Input: part model. Units: mm. Frame: model coordinates. A direction names the side the tool comes from. Round coordinates to 2 decimals unless told otherwise and drop trailing zeros. Loops run counter-clockwise (first coordinate to the right, second up) from the corner with the lowest first, then second, coordinate; pieces in that order, holes last. Notation, with made-up numbers: (75, 74) -> (115, 74) arc R36 ccw to (115, 110) -> close; hole circle Ø3 at (55, 13). An arc over 180 degrees is marked (long way). Answer as a JSON object with one key per item and string values.
```python
from build123d import *

# Parameters (mm, degrees)
SKETCH1_R           = 10
BOSS_EXTRUDE1_DEPTH = 187.5
SKETCH3_R           = 12.5
CUT_EXTRUDE1_START  = -13.5000001
SKETCH4_W           = 4
SKETCH4_H           = 6
CUT_EXTRUDE1_DEPTH  = 23.5000001


with BuildPart() as part:
    # Sketch1 → Boss-Extrude1 (new body, symmetric)
    with BuildSketch(Plane(origin=(0, 0, 0), x_dir=(0, 0, -1), z_dir=(1, 0, 0))):
        Circle(SKETCH1_R)
    extrude(amount=BOSS_EXTRUDE1_DEPTH, both=True)

    # Sketch3 → Loft1 section 0
    with BuildSketch(Plane(origin=(187.5, 0, 0), x_dir=(0, 0, -1), z_dir=(1, 0, 0)), mode=Mode.PRIVATE) as loft1_s0:
        Circle(SKETCH3_R)
    loft1 = loft([Vertex(197.5, 0, 0), loft1_s0.sketch])

    # Mirror1: Loft1 across plane
    add(loft1.mirror(Plane(origin=(0, 0, 0), x_dir=(0, 0, 1), z_dir=(1, 0, 0))))

    # Sketch4 → Cut-Extrude1 (cut)
    with BuildSketch(Plane.XY.offset(CUT_EXTRUDE1_START)):
        with Locations((196.492262498, 0)):
            Rectangle(SKETCH4_W, SKETCH4_H)
    cut_extrude1 = extrude(amount=CUT_EXTRUDE1_DEPTH, mode=Mode.SUBTRACT)

    # Mirror2: Cut-Extrude1 across plane
    add(cut_extrude1.mirror(Plane(origin=(0, 0, 0), x_dir=(0, 0, 1), z_dir=(1, 0, 0))), mode=Mode.SUBTRACT)


solid = part.part
```
1) Contact query for flat-ended pins moving along their axis: P1, Ø3, axis at y = -0.5, z = 1, coming from the -X side; P2, Ø3, axis at x = -27.5, y = -5, coming from the -Z side; P3, Ø7.5, axis at y = -5.5, z = 6, coming from the -X side. Output: stop coordinate, or through.
Output:
{"P1": "stops at x = -194.49", "P2": "stops at z = -9.37", "P3": "stops at x = -193.99"}
2) Reachability of faces 4 (the face through (-194.492, 0, 0)), 5 (the face through (187.5, 10.2, 0.1)), 6 (the face through (194.6, -3.2, -1.7)) from +Z, -Z, +X, -X, +Y, -Y: full face, straight path, thin tool, end or side. Return the list, or none.
Output:
{"face 4": "+Z, -Z, -X", "face 5": "none", "face 6": "+X"}
3) Section A-A, the plane x = 74. Output: boundary loops of the cut face in (y, z).
Output:
{"outline": "circle Ø20 at (0, 0)"}
4) Draft query along X for faces 1 (the face through (-194.6, -3.2, -1.7)), 2 (the face through (2.62, -9.76, 2.17)), 3 (the face through (194.492, 0, 0)). Return one class per face: +X half, -X half, draft (parallel to the pull), parting line (faces both ways), or undercut.
Output:
{"face 1": "-X half", "face 2": "undercut", "face 3": "+X half"}
5) Ray query, probe 1 along X at (y, z) = (10.5, 4); probe 2 along X at (y, z) = (-0.25, -10.5); probe 3 along Y at (x, z) = (-150, -0.75). Return the intervals inside material, ascending.
Output:
{"probe 1": "x = -188.51 to -187.5, 187.5 to 188.51", "probe 2": "x = -189.1 to -187.5, 187.5 to 189.1", "probe 3": "y = -9.97 to 9.97"}
